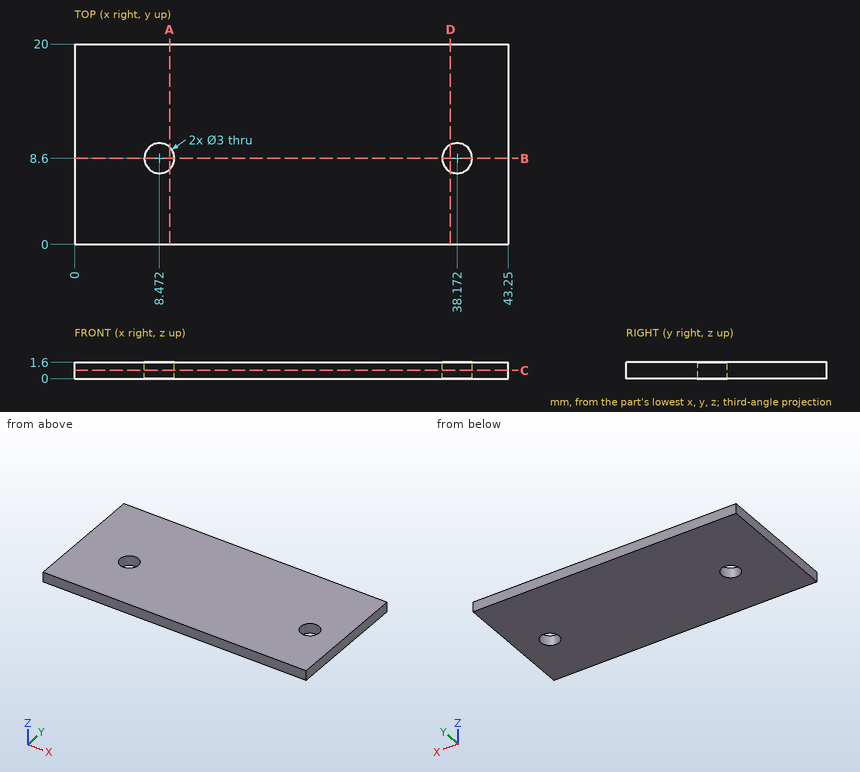
Print and shaded views of the part. All mm, measured from the part's lowest x, y and z. Coordinates: 2 decimals unless noted, no trailing zeros. Loops run counter-clockwise (first coordinate to the right, second up) from the corner with the lowest first, then second, coordinate; pieces in that order, holes last. Notation, with made-up numbers: M 38,56 L 93,56 A29 ccw 93,84 Z; hole C -40,71 d5. An arc over 180 degrees is marked long. Use a Markdown table: item, result. Add a question column.
Q1. Cut at C-C (z = 0.8). Write the cut outline in (x, y), and give its area (3 significant figures).
Q2. Probe L1, parallel to X at y = 8.6, z = 0.85. List the from-to ranges inside material, lowest first.
Q3. Pin check, flat tip, straight feed: P1, Ø2.5, axis at x = 38.17, y = 8.6, coming from the +Z side. Stop position of the tip, or through.
Q4. Cut at B-B (y = 8.6). Write the cut outline in (x, z).
Q5. Cut at D-D (x = 37.5). Write the cut outline in (y, z).
Q6. Cut at A-A (x = 9.5). Write the cut outline in (y, z), and give its area (3 significant figures).
Worked out:
| question | item | result |
|---|---|---|
| 1 | outline | M 0,0 L 43.25,0 L 43.25,20 L 0,20 Z; hole C 8.47,8.6 d3; hole C 38.17,8.6 d3 |
| 1 | area | 851 mm2 |
| 2 | L1 | x = 0 to 6.97, 9.97 to 36.67, 39.67 to 43.25 |
| 3 | P1 | passes through |
| 4 | outline | M 0,0 L 6.97,0 L 6.97,1.6 L 0,1.6 Z; M 9.97,0 L 36.67,0 L 36.67,1.6 L 9.97,1.6 Z; M 39.67,0 L 43.25,0 L 43.25,1.6 L 39.67,1.6 Z |
| 5 | outline | M 0,0 L 7.26,0 L 7.26,1.6 L 0,1.6 Z; M 9.94,0 L 20,0 L 20,1.6 L 9.94,1.6 Z |
| 6 | outline | M 0,0 L 7.51,0 L 7.51,1.6 L 0,1.6 Z; M 9.69,0 L 20,0 L 20,1.6 L 9.69,1.6 Z |
| 6 | area | 28.5 mm2 |
